Read the model definition and answer for the solid it produces. Units are mm, in the model's axes. Give positions to 0.01 mm unless a question says otherwise; leave off trailing zeros. Put each result on its own line as item: value. Start each with the question number.
1. A cutting plane is placed at A-A, the plane y = -260.5. Count the separate pieces of the cut face and the enclosed holes in it, plus the area to 3 significant figures.
2. For a pull along X with two mould halves and no side action, classify faces 1 (the flat face through (0, -187, 12.75)), 2 (the flat face through (-15, -187, -2)), 3 (the flat face through (9, -187, -7.5)) as released by +X, released by -X, zero draft, split by the parting line, or undercut.
3. Consider L1, parallel to X at y = -124, z = -3; L2, parallel to Z at x = 10.25, y = -276; L3, parallel to Z at x = 13, y = -139.5. Determine where each line is inside the solid, lowest interval first. Write a range as from..to.
4. Given pin 1 Ø1.5 at (x, y) = (1, -306) entering from -Z, flat-ended and moving along its own axis, determine where the tip first touches the part or whether it passes through.
```python
from build123d import *

# Parameters (mm, degrees)
SKETCH1_R           = 2.5
SKETCH1_W           = 3.5
SKETCH1_H           = 3.5
BOSS_EXTRUDE1_DEPTH = 380
FILLET1_R           = 1


with BuildPart() as part:
    # Sketch1 → Boss-Extrude1 (new body)
    with BuildSketch(Plane(origin=(0, 0, 0), x_dir=(1, 0, 0), z_dir=(0, 1, 0))):
        Polygon((-15, 7.5), (-15, -4.5), (-12, -4.5), (-12, -2), (-13.5, -2), (-13.5, 0.5), (-10, 0.5), (-5.25, -4.25), (-5.25, -10.75), (-10, -15.5), (-13.5, -15.5), (-13.5, -13), (-12, -13), (-12, -10.5), (-15, -10.5), (-15, -22.5), (-3, -22.5), (-3, -19.5), (-5.5, -19.5), (-5.5, -21), (-8, -21), (-8, -17.5), (-3.25, -12.75), (3.25, -12.75), (8, -17.5), (8, -21), (5.5, -21), (5.5, -19.5), (3, -19.5), (3, -22.5), (15, -22.5), (15, -10.5), (12, -10.5), (12, -13), (13.5, -13), (13.5, -15.5), (10, -15.5), (5.25, -10.75), (5.25, -4.25), (10, 0.5), (13.5, 0.5), (13.5, -2), (12, -2), (12, -4.5), (15, -4.5), (15, 7.5), (3, 7.5), (3, 4.5), (5.5, 4.5), (5.5, 6), (8, 6), (8, 2.5), (3.25, -2.25), (-3.25, -2.25), (-8, 2.5), (-8, 6), (-5.5, 6), (-5.5, 4.5), (-3, 4.5), (-3, 7.5), align=None)
        with Locations(Location((0, -7.5, 0), (0, 0, 270))):
            Circle(SKETCH1_R, mode=Mode.SUBTRACT)
        with Locations((-11.5, 4)):
            Rectangle(SKETCH1_W, SKETCH1_H, mode=Mode.SUBTRACT)
        with Locations((11.5, 4)):
            Rectangle(SKETCH1_W, SKETCH1_H, mode=Mode.SUBTRACT)
        with Locations((11.5, -19)):
            Rectangle(SKETCH1_W, SKETCH1_H, mode=Mode.SUBTRACT)
        with Locations((-11.5, -19)):
            Rectangle(SKETCH1_W, SKETCH1_H, mode=Mode.SUBTRACT)
    extrude(amount=-BOSS_EXTRUDE1_DEPTH)

    # Fillet1
    fillet1_edges = [part.edges().sort_by_distance(p)[0] for p in [
        (15, -190, 10.5),
        (15, -190, 22.5),
        (3, -190, 22.5),
        (-3, -190, 22.5),
        (-15, -190, 22.5),
        (-15, -190, 10.5),
        (-15, -190, 4.5),
        (-15, -190, -7.5),
        (-3, -190, -7.5),
        (3, -190, -7.5),
        (15, -190, -7.5),
        (15, -190, 4.5),
    ]]
    fillet(fillet1_edges, radius=FILLET1_R)


solid = part.part
```
Return value:
1. separate pieces: 1
1. enclosed holes: 5
1. area: 385 mm2
2. face 1: undercut
2. face 2: released by -X
2. face 3: zero draft
3. L1: x = -15..-13.25, -9.75..-8, 8..9.75, 13.25..15
3. L2: z = -7.5..-5.75, -2.25..-0.5, 15.5..17.25, 20.75..22.5
3. L3: z = -7.5..-5.75, -2.25..-0.5, 2..4.5, 10.5..13, 15.5..17.25, 20.75..22.5
4. pin 1: stops at z = 2.25
